Autodesk Inventor part; units mm, degrees
ref_plane "YZ Plane" through (0, 0, 0) normal (1, 0, 0) x (0, 1, 0)
ref_plane "XZ Plane" through (0, 0, 0) normal (0, 1, 0) x (-1, 0, 0)
ref_plane "XY Plane" through (0, 0, 0) normal (0, 0, 1) x (1, 0, 0)
sketch "Sketch1" plane through (0, 0, 0) normal (0, 0, 1) x (1, 0, 0)
  line L0 (0, 0) -> (254, 0)
  line L1 (254, 0) -> (254, 139.7)
  line L2 (254, 139.7) -> (0, 139.7)
  line L3 (0, 139.7) -> (0, 0)
  dimension "d0" = 254
  dimension "d1" = 139.7
extrude "Extrusion1" add sketch "Sketch1" along normal blind 177.8
sketch "Sketch4" plane through (254, 0, 0) normal (1, 0, 0) x (0, 0, -1)
  line L0 (-177.8, 139.7) -> (-177.8, 0)
  line L1 (0, 0) -> (-177.8, 0)
  line L2 (0, 139.7) -> (-177.8, 139.7)
  line L3 (-177.8, 139.7) -> (-177.8, 3.175)
  line L4 (-177.8, 3.175) -> (-152.4, 3.175)
  line L5 (-152.4, 3.175) -> (0, 139.7)
  dimension "d10" = 3.175
  dimension "d11" = 25.4
extrude "Extrusion3" cut sketch "Sketch4" against normal through all
sketch "Sketch5" plane through (0, 0, 0) normal (0, 0, -1) x (-1, 0, 0)
  line L0 (0, 0) -> (-254, 0)
  line L1 (0, 139.7) -> (0, 0)
  line L2 (-254, 139.7) -> (-228.6, 139.7)
  line L3 (-228.6, 139.7) -> (-228.6, 3.175)
  line L4 (-228.6, 3.175) -> (-254, 3.175)
  line L5 (-254, 3.175) -> (-254, 139.7)
  line L6 (0, 139.7) -> (-25.4, 139.7)
  line L7 (-25.4, 139.7) -> (-25.4, 3.175)
  line L8 (-25.4, 3.175) -> (0, 3.175)
  line L9 (0, 3.175) -> (0, 139.7)
  dimension "d15" = 3.175
  dimension "d16" = 25.4
extrude "Extrusion4" cut sketch "Sketch5" against normal through all
shell "Shell1" thickness 3.175 removed faces 2 at (160.8667, 48.6833, 0) at (84.6667, 0, 59.2667)
properties part number "Panel_ShooterShroud" material "Polycarbonate, Smoke"
The model under review builds one solid part; all positions refer to its coordinate system, in mm. A direction names the side the tool comes from. Round coordinates to 2 decimals unless told otherwise and drop trailing zeros. Loops run counter-clockwise (first coordinate to the right, second up) from the corner with the lowest first, then second, coordinate; pieces in that order, holes last. Notation, with made-up numbers: M 40.5,78 L 74.5,78 A35 ccw 74.5,116 Z; hole C 53,15.5 d11. An arc over 180 degrees is marked long. Write item = value, one per line.
Item 1: Take a section at B-B on z = 122.5. Write out the cut boundary in (x, y) (3 decimals), then the cut area to 3 significant figures.
Return value:
outline = M 0,0 L 28.575,0 L 28.575,25.698 L 225.425,25.698 L 225.425,0 L 254,0 L 254,3.175 L 228.6,3.175 L 228.6,29.96 L 25.4,29.96 L 25.4,3.175 L 0,3.175 Z
area = 1,190 mm2
Item 2: Insertion check: P1, Ø4, axis at x = 186.5, z = 99.5, coming from the +Y side; P2, Ø4, axis at x = 161.5, z = 32.5, coming from the +Y side; P3, Ø12, axis at x = 105, y = 17.5, coming from the +Z side. Each pin has a flat end and moves straight along its axis. Give the tip position at first contact, or say it passes through.
Return value:
P1 = 52.36
P2 = 112.38
P3 = 143.11
Item 3: Take a section at C-C on x = 40. Write out the cut boundary in (y, z) (3 decimals), then the cut area to 3 significant figures.
Return value:
outline = M 0,151.186 L 135.437,0 L 139.7,0 L 3.175,152.4 L 3.175,177.8 L 0,177.8 Z
area = 730 mm2
Item 4: Machinability: for faces 1 (the flat face through (28.575, 54, 58)), 2 (the flat face through (228.6, 42, 41)), 3 (the flat face through (126, 137, 0)), which of the approach directions +Z, -Z, +X, -X, +Y, -Y give a long, thin tool a straight path to every point of the face, cutting with its end or side? Answer none if there is none.
Return value:
face_1 = -Z, -Y
face_2 = +Z, -Z, +X, +Y
face_3 = -Z, +X, -X, +Y, -Y
Item 5: For line 1 (X direction, y = 50, z = 27) (3 decimals); line 2 (Y direction, x = 55, z = 164) (3 decimals); line 3 (X direction, y = 114.5, z = 25.5), list the stretches that pass through material, from the lowest coordinate up. Write a range as [from, to].
Return value:
line_1 = [25.4, 28.575], [225.425, 228.6]
line_2 = [0, 3.175]
line_3 = [25.4, 228.6]
Item 6: Take a section at A-A on y = 95.5. Write out the cut boundary in (x, z) (3 decimals), then the cut area to 3 significant figures.
Return value:
outline = M 25.4,0 L 28.575,0 L 28.575,44.581 L 225.425,44.581 L 225.425,0 L 228.6,0 L 228.6,49.34 L 25.4,49.34 Z
area = 1,250 mm2
Item 7: The part is to be moulded in two halves that separate along X. For faces 4 (the flat face through (118, 3.175, 155)), 5 (the flat face through (128.38, 66.77, 76.65)), 6 (the flat face through (25.4, 42, 41)), say which applies: released by +X, released by -X, zero draft, split by the parting line, or undercut.
Return value:
face_4 = zero draft
face_5 = undercut
face_6 = released by -X
Item 8: Take a section at D-D on y = 63. Write out the cut boundary in (x, z) (3 decimals), then the cut area to 3 significant figures.
Return value:
outline = M 25.4,0 L 28.575,0 L 28.575,80.86 L 225.425,80.86 L 225.425,0 L 228.6,0 L 228.6,85.619 L 25.4,85.619 Z
area = 1,480 mm2
